Could you check a few things on this drawing? It's one solid part, dimensions in mm from its lowest x, y, z. A direction names the side the tool comes from. Coordinates: 2 decimals unless noted, no trailing zeros. Order: outer loops, then holes, each group sorted by start corner. A loop starts at its lowest first (then second) coordinate and runs counter-clockwise, first axis right, second up. Notation, with made-up numbers: (77.5, -32.75) - (119.5, -32.75) arc R5 ccw to (119.5, -28.75) - close; hole circle Ø9 at (72, 82.5). An arc over 180 degrees is marked (long way). Answer in a Markdown table with one row per item. Add a question column.
Item 1: I want a section at B-B (z = 32). Please give me the cut outline in (x, y) (1 decimal).
Item 2: I want a section at C-C (y = 23.5). Please give me the cut outline in (x, z).
Item 3: I want a section at A-A (x = 18.55). Please give me the cut outline in (y, z), plus the area to 3 significant figures.
Item 4: On a 3-axis mill with a long thin cutter (end or side, diameter ignored), from which of +Z, -Z, +X, -X, +Y, -Y can I reach the whole of each face in a straight line? I mean the marked faces 4, 5 and 6. Say none if no direction works.
Item 5: Will these pins go through, and if not, where does the flat tip stop? pin 1 Ø1.7 at (x, y) = (17.5, 47.5) entering from +Z; pin 2 Ø4 at (x, y) = (26, 41.5) entering from +Z (1 decimal); pin 3 Ø8 at (y, z) = (19, 29) entering from +X; pin 4 Ø3 at (x, y) = (29, 41.5) entering from +Z.
Item 6: If I drill on line 1 along Y through (x, z) = (18, 24); line 2 along Z through (x, y) = (18.5, 9.5); line 3 along Z through (x, y) = (20, 18), over which ranges is the centre line in solid material (lowest first)? Write a range as from..to.
Item 7: Thinking about a two-plate mould opening in Y: for the marked faces 1, 2 and 3, which applies, +Y half, -Y half, draft (parallel to the pull), parting line (faces both ways), or undercut?
Item 8: I want a section at D-D (x = 32). Please give me the cut outline in (y, z) (1 decimal).
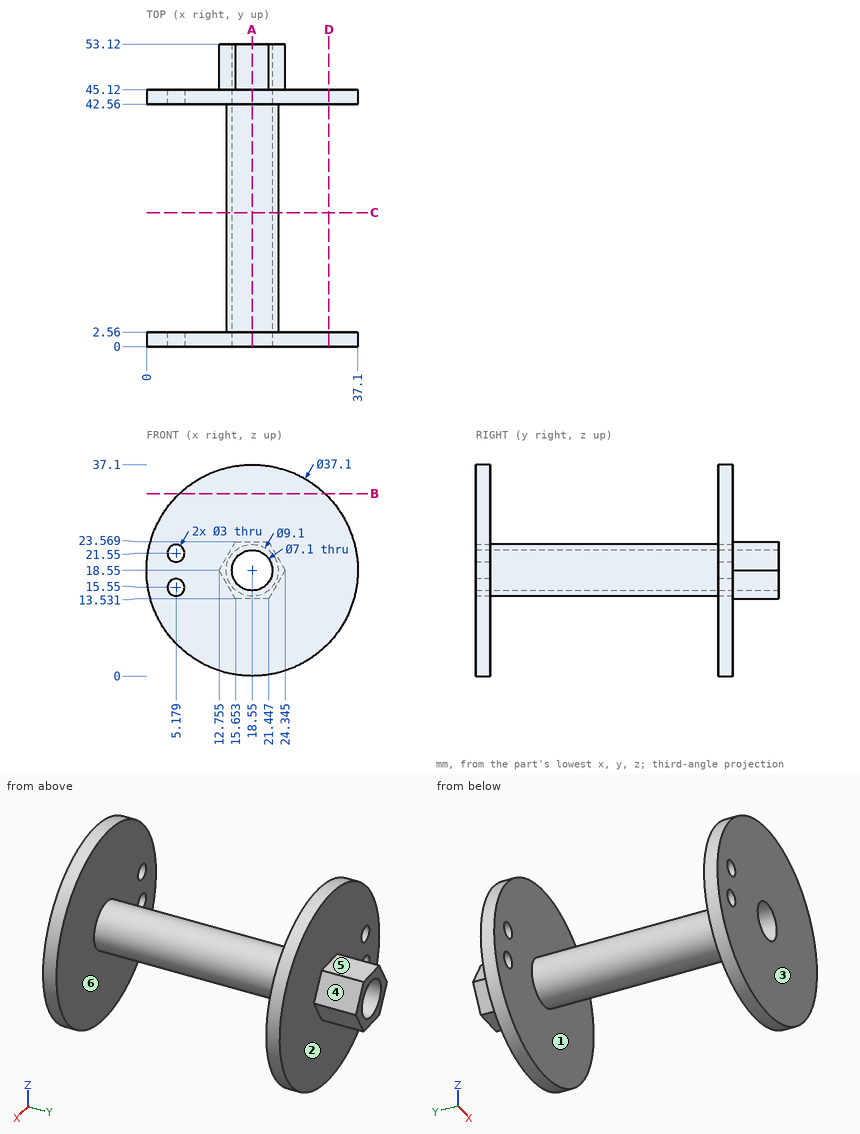
Values follow:
| question | item | result |
|---|---|---|
| 1 | outline | (5.8, 0) - (31.3, 0) - (31.3, 2.6) - (5.8, 2.6) - close; (5.8, 42.6) - (31.3, 42.6) - (31.3, 45.1) - (5.8, 45.1) - close |
| 2 | outline | circle Ø9.1 at (18.55, 18.55); hole circle Ø7.1 at (18.55, 18.55) |
| 3 | outline | (0, 0) - (2.56, 0) - (2.56, 14) - (42.56, 14) - (42.56, 0) - (45.12, 0) - (45.12, 13.53) - (53.12, 13.53) - (53.12, 15) - (0, 15) - close; (0, 22.1) - (53.12, 22.1) - (53.12, 23.57) - (45.12, 23.57) - (45.12, 37.1) - (42.56, 37.1) - (42.56, 23.1) - (2.56, 23.1) - (2.56, 37.1) - (0, 37.1) - close |
| 3 | area | 257 mm^2 |
| 4 | face 4 | +Z, +X, +Y |
| 4 | face 5 | +Z, +X, -X, +Y |
| 4 | face 6 | none |
| 5 | pin 1 | stops at z = 23.57 |
| 5 | pin 2 | stops at z = 36.2 |
| 5 | pin 3 | passes through |
| 5 | pin 4 | stops at z = 34.55 |
| 6 | line 1 | y = 0..2.56, 42.56..45.12 |
| 6 | line 2 | z = 14..15, 22.1..23.1 |
| 6 | line 3 | z = 14.24..15.31, 21.79..22.86 |
| 7 | face 1 | undercut |
| 7 | face 2 | +Y half |
| 7 | face 3 | -Y half |
| 8 | outline | (0, 5.8) - (2.6, 5.8) - (2.6, 31.3) - (0, 31.3) - close; (42.6, 5.8) - (45.1, 5.8) - (45.1, 31.3) - (42.6, 31.3) - close |
